For this review, use the dimensioned drawing (mm, ordinates from the lowest corner) and the shaded views. A direction names the side the tool comes from. Round coordinates to 2 decimals unless told otherwise and drop trailing zeros. Write each loop counter-clockwise with the first axis right and the second up, starting at its lowest first coordinate (ties: lowest second). Pieces come first, ordered by that corner, then holes. Notation, with made-up numbers: (84.25, 66) -> (111.25, 66) arc R17 cw to (111.25, 85) -> close; hole circle Ø5 at (-12.75, 68). An arc over 180 degrees is marked (long way). Answer as CSV lines item,"result". Start each with the question number.
Item 1: For pin 1 Ø3 at (y, z) = (32, 2) entering from -X; pin 2 Ø2.5 at (x, y) = (4.63, 4.63) entering from +Z; pin 3 Ø5 at (x, z) = (14.5, 2) entering from +Y; pin 4 Ø3 at (x, y) = (13, 30.5) entering from -Z, all flat-tipped, find the tip position at first contact; note any pin that passes through.
Item 2: Machinability: for the marked faces 5 and 6, which of the approach directions +Z, -Z, +X, -X, +Y, -Y give a long, thin tool a straight path to every point of the face, cutting with its end or side? Answer none if there is none.
Item 3: Wall thickness on probe 1 along Y at (x, z) = (29, 9.75) (1 decimal); probe 2 along X at (y, z) = (28.5, 1.5) (1 decimal); probe 3 along Y at (x, z) = (17.5, 6.5): over which ranges is each line inside the solid? List them lowest first. Write a range as from..to.
Item 4: Take a section at A-A on y = 3. Give the boundary of the cut face in (x, z) (1 decimal).
Item 5: Mouldability with a two-part tool opening along Y and no side actions: class the marked faces 1, 2, 3 and 4 as +Y half, -Y half, draft (parallel to the pull), parting line (faces both ways), or undercut.
Item 6: Take a section at C-C on y = 25. Give the boundary of the cut face in (x, z) (1 decimal), then the cut area to 3 significant figures.
Item 7: Take a section at D-D on z = 4.25. Count the separate pieces of the cut face and the enclosed holes in it.
Item 8: Take a section at B-B on x = 15.5. Give the boundary of the cut face in (y, z).
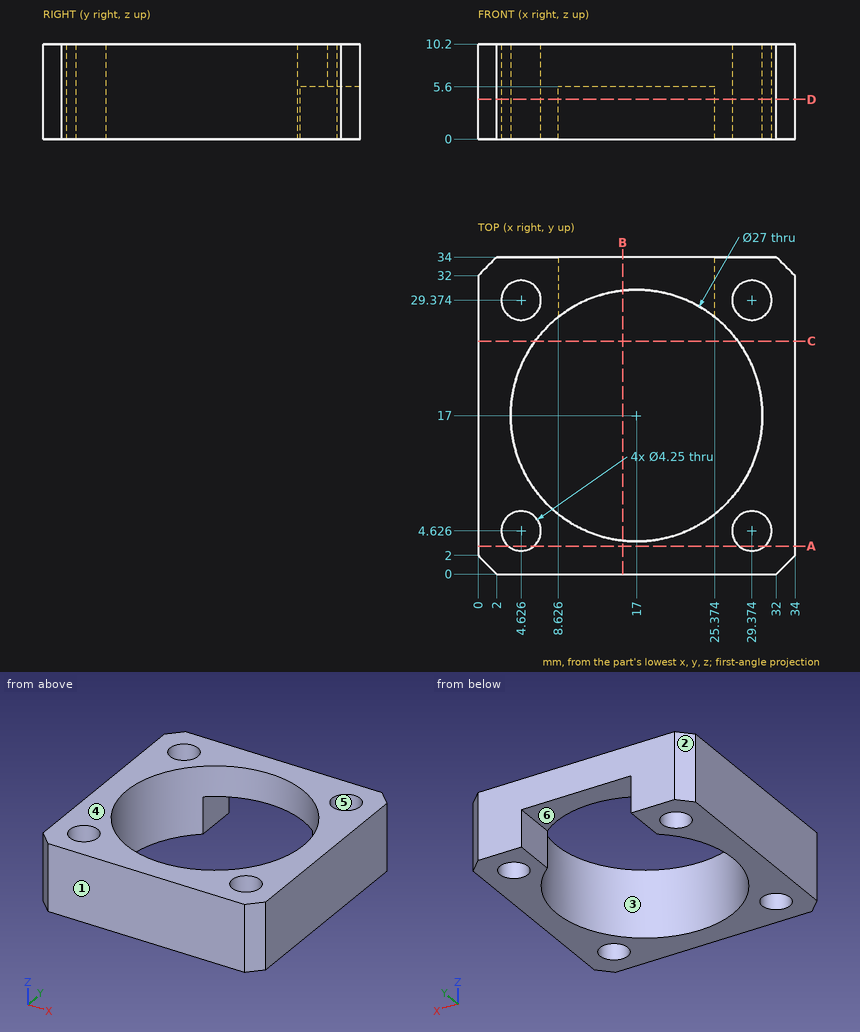
Output values:
1,pin 1,"stops at x = 0"
1,pin 2,"passes through"
1,pin 3,"stops at y = 4.46"
1,pin 4,"stops at z = 5.6"
2,face 5,"+Z, -Z"
2,face 6,"-Z, +Y"
3,probe 1,"y = 0..2.5, 6.7..10.8, 23.2..27.3, 31.5..34"
3,probe 2,"x = 0..2.7, 6.6..8.6, 25.4..27.4, 31.3..34"
3,probe 3,"y = 0..3.51, 30.49..34"
4,outline,"(0, 0) -> (3.3, 0) -> (3.3, 10.2) -> (0, 10.2) -> close; (6, 0) -> (28, 0) -> (28, 10.2) -> (6, 10.2) -> close; (30.7, 0) -> (34, 0) -> (34, 10.2) -> (30.7, 10.2) -> close"
5,face 1,"-Y half"
5,face 2,"+Y half"
5,face 3,"undercut"
5,face 4,"draft"
6,outline,"(0, 0) -> (6.1, 0) -> (6.1, 10.2) -> (0, 10.2) -> close; (27.9, 0) -> (34, 0) -> (34, 10.2) -> (27.9, 10.2) -> close"
6,area,"125 mm^2"
7,separate pieces,"1"
7,enclosed holes,"4"
8,outline,"(0, 0) -> (3.58, 0) -> (3.58, 10.2) -> (0, 10.2) -> close; (30.42, 5.6) -> (34, 5.6) -> (34, 10.2) -> (30.42, 10.2) -> close"
